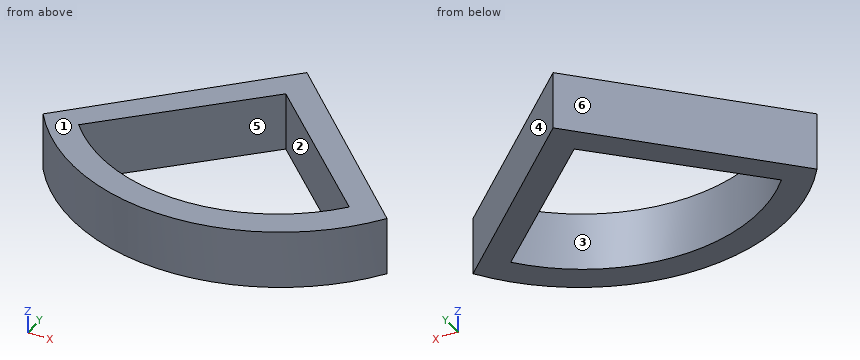
```python
from build123d import *

# Parameters (mm, degrees)
F1_DEPTH = 25.4
F3_DEPTH = 25.4
F5_DEPTH = 25.4


with BuildPart() as f1:
    # F0 (on Top) → F1 (new body)
    with BuildSketch(Plane.XY):
        with BuildLine():
            Line((75.73466, 0), (0, 73.902369))
            Line((0, 73.902369), (-74.818514, 0))
            ThreePointArc((-74.818514, 0), (0.458073, -39.399989), (75.73466, 0))
        make_face()
    extrude(amount=F1_DEPTH)

    # F2 (on Top) → F3 (cut)
    with BuildSketch(Plane.XY):
        with BuildLine():
            Line((63.833756, 0), (0, 62.908627))
            Line((0, 62.908627), (-62.168982, -0.174606))
            ThreePointArc((-62.168982, -0.174606), (0.876457, -31.889673), (63.833756, 0))
        make_face()
    extrude(amount=-F3_DEPTH, mode=Mode.SUBTRACT)

    # F4 (on Top) → F5 (cut)
    with BuildSketch(Plane.XY):
        with BuildLine():
            Line((59.217848, 0), (0, 57.106376))
            Line((0, 57.106376), (-59.244044, 0))
            ThreePointArc((-59.244044, 0), (-0.013098, -27.205963), (59.217848, 0))
        make_face()
    extrude(amount=F5_DEPTH, mode=Mode.SUBTRACT)


solid = f1.part
```
Read the model definition and answer for the solid it produces. Units are mm, in the model's axes. Face numbers are marked on the shaded views. A direction names the side the tool comes from. Coordinates: 2 decimals unless noted, no trailing zeros. Loops run counter-clockwise (first coordinate to the right, second up) from the corner with the lowest first, then second, coordinate; pieces in that order, holes last. Notation, with made-up numbers: (10.5, 32) -> (57.5, 32) arc R20 ccw to (57.5, 55) -> close; hole circle Ø11 at (-24.5, -1.5). An arc over 180 degrees is marked (long way). Return JSON: item names as keys, results as strings.
Item 1: Find the intervals of material crossed by probe 1 along X at (y, z) = (50.5, 10); probe 2 along X at (y, z) = (47, 14.25); probe 3 along Y at (x, z) = (-15, 19.75), in increasing order.
Answers:
{"probe 1": "x = -23.69 to -6.85, 6.85 to 23.98", "probe 2": "x = -27.24 to -10.48, 10.48 to 27.57", "probe 3": "y = -38.09 to -25.75, 42.65 to 59.09"}
Item 2: For a pull along Y with two mould halves and no side action, classify the marked faces 1, 2, 3 and 4 as +Y half, -Y half, draft (parallel to the pull), parting line (faces both ways), or undercut.
Answers:
{"face 1": "draft", "face 2": "undercut", "face 3": "undercut", "face 4": "+Y half"}
Item 3: Find section D-D (x = 63). Determine the outline of the cut face in (y, z).
Answers:
{"outline": "(-14.73, 0) -> (12.43, 0) -> (12.43, 25.4) -> (-14.73, 25.4) -> close"}
Item 4: Find section B-B (y = 45). Determine the outline of the cut face in (x, z), plus the area to 3 significant figures.
Answers:
{"outline": "(-29.26, 0) -> (-12.56, 0) -> (-12.56, 25.4) -> (-29.26, 25.4) -> close; (12.55, 0) -> (29.62, 0) -> (29.62, 25.4) -> (12.55, 25.4) -> close", "area": "858 mm2"}
Item 5: For the marked faces 5 and 6, determine the directions among +Z, -Z, +X, -X, +Y, -Y from which every point of the face is accessible in a straight line to the end or side of a thin tool.
Answers:
{"face 5": "+Z, -Z", "face 6": "+Z, -Z, -X, +Y"}
Item 6: Find section C-C (z = 6.75). Determine the outline of the cut face in (x, y).
Answers:
{"outline": "(-74.82, 0) arc R91.61 ccw to (75.73, 0) -> (0, 73.9) -> close; hole (-59.24, 0) arc R78.08 ccw to (59.22, 0) -> (0, 57.11) -> close"}
Item 7: Flat-ended cylindrical pins translate along their axes: P1, Ø12, axis at x = -55, z = 14.5, coming from the +Y side; P2, Ø6, axis at y = 57.5, z = 3, coming from the -X side; P3, Ø8, axis at y = 13.5, z = 16.5, coming from the -X side. Find the tip coordinate at first contact, or state that the pin passes through.
Answers:
{"P1": "stops at y = 25.5", "P2": "stops at x = -19.64", "P3": "stops at x = -65.2"}
Item 8: Find section A-A (x = 13). Determine the outline of the cut face in (y, z), plus the area to 3 significant figures.
Answers:
{"outline": "(-38.54, 0) -> (-26.11, 0) -> (-26.11, 25.4) -> (-38.54, 25.4) -> close; (44.57, 0) -> (61.22, 0) -> (61.22, 25.4) -> (44.57, 25.4) -> close", "area": "738 mm2"}
